from build123d import *

# Parameters (mm, degrees)
SKETCH1_W                   = 18
SKETCH1_H                   = 18
BOSS_EXTRUDE1_DEPTH         = 35
SKETCH5_W                   = 13
SKETCH5_H                   = 13
CUT_EXTRUDE1_DEPTH          = 30
CUT_EXTRUDE3_REACH          = 45.278
SKETCH7_W                   = 10.5
SKETCH7_H                   = 20
SKETCH8_W                   = 18
SKETCH8_H                   = 18
BOSS_EXTRUDE2_DEPTH         = 10
SKETCH9_W                   = 11.43
SKETCH9_H                   = 5.85
CUT_EXTRUDE4_DEPTH          = 44.278170017
F_1_4_CLEARANCE_HOLE1_D     = 7.14248
F_1_4_CLEARANCE_HOLE1_DEPTH = 15
F_1_4_CLEARANCE_HOLE1_TIP   = 2.145817477
CUT_EXTRUDE5_REACH          = 45.278
SKETCH12_W                  = 10
SKETCH12_H                  = 20


with BuildPart() as part:
    # Sketch1 → Boss-Extrude1 (new body)
    with BuildSketch(Plane(origin=(0, 0, 0), x_dir=(1, 0, 0), z_dir=(0, 1, 0))):
        with Locations((9, 9)):
            Rectangle(SKETCH1_W, SKETCH1_H)
    extrude(amount=BOSS_EXTRUDE1_DEPTH)

    # Sketch5 → Cut-Extrude1 (cut)
    with BuildSketch(Plane(origin=(0, 35, 0), x_dir=(1, 0, 0), z_dir=(0, 1, 0))):
        with Locations((9, 9)):
            Rectangle(SKETCH5_W, SKETCH5_H)
    extrude(amount=-CUT_EXTRUDE1_DEPTH, mode=Mode.SUBTRACT)

    # Sketch7 → Cut-Extrude3 (cut, up to next)
    with BuildSketch(Plane(origin=(18, 0, 0), x_dir=(0, 0, -1), z_dir=(1, 0, 0)), mode=Mode.PRIVATE) as cut_extrude3_sk1:
        with Locations((9.25, 20)):
            Rectangle(SKETCH7_W, SKETCH7_H)
    cut_extrude3_tool1 = extrude(cut_extrude3_sk1.sketch, amount=-CUT_EXTRUDE3_REACH, mode=Mode.PRIVATE) & part.part
    add(cut_extrude3_tool1.solids().sort_by_distance((18, 20, -9.25))[0], mode=Mode.SUBTRACT)

    # Sketch8 → Boss-Extrude2 (add)
    with BuildSketch(Plane.XZ):
        with Locations((9, -9)):
            Rectangle(SKETCH8_W, SKETCH8_H)
    extrude(amount=BOSS_EXTRUDE2_DEPTH)

    # Sketch9 → Cut-Extrude4 (cut, through all)
    with BuildSketch(Plane.XY):
        with Locations((9, -2.5)):
            Rectangle(SKETCH9_W, SKETCH9_H)
    extrude(amount=-CUT_EXTRUDE4_DEPTH, mode=Mode.SUBTRACT)

    # 1/4 Clearance Hole1
    with Locations(Plane(origin=(0, -10, 0), x_dir=(-1, 0, 0), z_dir=(0, -1, 0))):
        with Locations((-9, 9)):
            Hole(F_1_4_CLEARANCE_HOLE1_D / 2, depth=F_1_4_CLEARANCE_HOLE1_DEPTH)
            with Locations((0, 0, -(F_1_4_CLEARANCE_HOLE1_DEPTH + F_1_4_CLEARANCE_HOLE1_TIP / 2))):  # 118° drill point
                Cone(0, F_1_4_CLEARANCE_HOLE1_D / 2, F_1_4_CLEARANCE_HOLE1_TIP, mode=Mode.SUBTRACT)

    # Sketch12 → Cut-Extrude5 (cut, up to next)
    with BuildSketch(Plane.XY, mode=Mode.PRIVATE) as cut_extrude5_sk1:
        with Locations((9.5, 20)):
            Rectangle(SKETCH12_W, SKETCH12_H)
    cut_extrude5_tool1 = extrude(cut_extrude5_sk1.sketch, amount=-CUT_EXTRUDE5_REACH, mode=Mode.PRIVATE) & part.part
    add(cut_extrude5_tool1.solids().sort_by_distance((9.5, 20, 0))[0], mode=Mode.SUBTRACT)


solid = part.part
Input: part model. Units: mm. Frame: model coordinates. A direction names the side the tool comes from. Give positions to 0.01 mm unless a question says otherwise; leave off trailing zeros. Write each loop counter-clockwise with the first axis right and the second up, starting at its lowest first coordinate (ties: lowest second). Pieces come first, ordered by that corner, then holes.
Q1. Section C-C, the plane z = -5. Output: boundary loops of the cut face in (x, y) (3 decimals), plus the area to 3 significant figures.
Q2. Pull-direction query (Y, two-part tool) for faces 1 (the face through (17, 35, -9)), 2 (the face through (18, 8, -9)), 3 (the face through (17, 20, -14.5)); classes: pulls with the +Y half, pulls with the -Y half, needs draft (parallel to the pull), parting line crosses it, or undercut.
Q3. Set-up query: faces 4 (the face through (15.5, 24, -3)), 5 (the face through (17, 30, -9)), 6 (the face through (0, 13, -9)), 7 (the face through (13, -5.425, -9)), 8 (the face through (14.5, 20, -1)). Return all of +Z, -Z, +X, -X, +Y, -Y with unobstructed straight access to the full face (end or side cutting, diameter ignored); none if empty.
Q4. Material intervals for probe 1 along Y at (x, z) = (11.25, -1.5) (3 decimals); probe 2 along X at (y, z) = (-9, -9); probe 3 along Y at (x, z) = (14.25, -4.5) (3 decimals), sorted ascending.
Q5. First-contact query: P1, Ø4, axis at x = 7, z = -9, coming from the +Y side. Flat tip, straight axial feed; report the tip coordinate or a pass-through.
Q6. Section D-D, the plane z = -1.75. Output: boundary loops of the cut face in (x, y) (3 decimals).
Q7. Section A-A, the plane y = 25. Output: boundary loops of the cut face in (x, z), plus the area to 3 significant figures.
Q8. Section B-B, the plane x = 16. Output: boundary loops of the cut face in (y, z).
Filled in:
1. outline: (0, -10) - (18, -10) - (18, 10) - (15.5, 10) - (15.5, 5) - (2.5, 5) - (2.5, 35) - (0, 35) - close; (15.5, 30) - (18, 30) - (18, 35) - (15.5, 35) - close; hole (3.285, -5.425) - (14.715, -5.425) - (14.715, 0.425) - (3.285, 0.425) - close
1. area: 303 mm2
2. face 1: pulls with the +Y half
2. face 2: needs draft
2. face 3: undercut
3. face 4: +Y
3. face 5: +X
3. face 6: +Z, -Z, -X, +Y, -Y
3. face 7: +Z, -Z
3. face 8: +Z
4. probe 1: y = -10 to -5.425, 0.425 to 10, 30 to 35
4. probe 2: x = 0 to 5.43, 12.57 to 18
4. probe 3: y = -10 to -5.425, 0.425 to 5
5. P1: stops at y = 5
6. outline: (0, -10) - (18, -10) - (18, 35) - (0, 35) - close; hole (3.285, -5.425) - (14.715, -5.425) - (14.715, 0.425) - (3.285, 0.425) - close; hole (4.5, 10) - (14.5, 10) - (14.5, 30) - (4.5, 30) - close
7. outline: (0, -18) - (18, -18) - (18, -14.5) - (15.5, -14.5) - (15.5, -15.5) - (2.5, -15.5) - (2.5, -2.5) - (4.5, -2.5) - (4.5, 0) - (0, 0) - close; (14.5, -2.5) - (15.5, -2.5) - (15.5, -4) - (18, -4) - (18, 0) - (14.5, 0) - close
7. area: 104 mm2
8. outline: (-10, -18) - (35, -18) - (35, 0) - (-10, 0) - close; hole (10, -14.5) - (30, -14.5) - (30, -4) - (10, -4) - close
